The figure shows three views and two pictorial views of one solid part (mm, origin at its lowest corner). Answer the questions. A direction names the side the tool comes from. Coordinates: 2 decimals unless noted, no trailing zeros. Write each loop counter-clockwise with the first axis right and the second up, starting at its lowest first coordinate (ties: lowest second). Pieces come first, ordered by that corner, then holes. Notation, with made-up numbers: M 21.25,52.5 L 37.25,52.5 A23 ccw 37.25,67.5 Z; hole C 35.5,-12.5 d3. An arc over 180 degrees is marked long. Use a Markdown table: item, result. Add a question column.
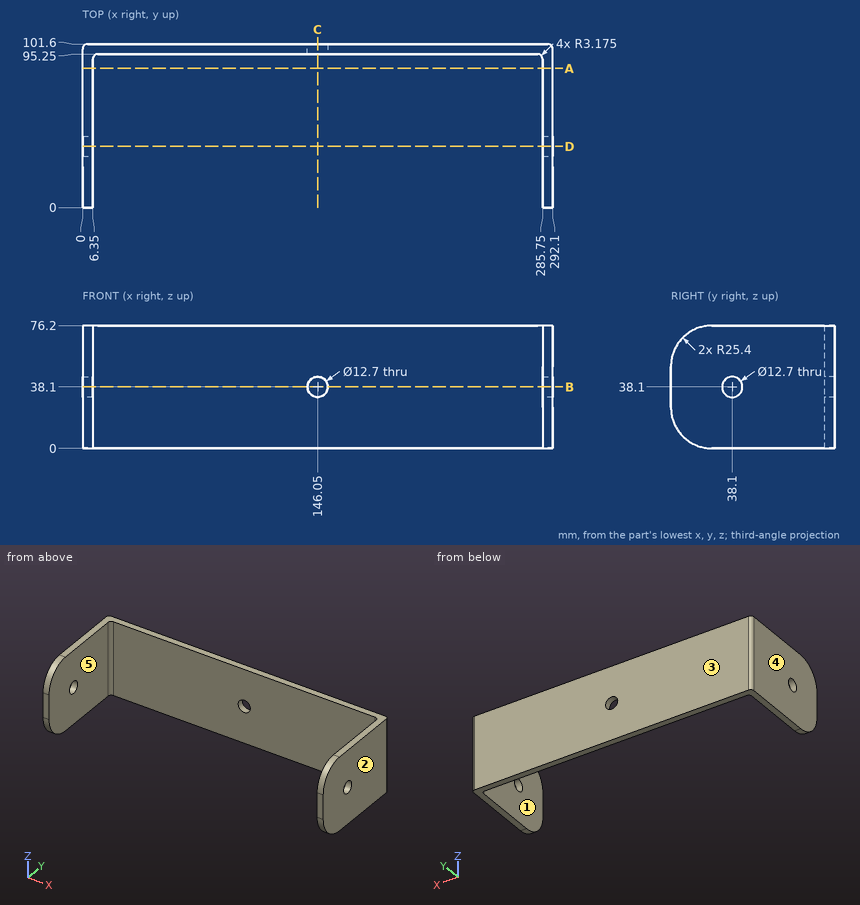
Item 1: Consider probe 1 along X at (y, z) = (92, 46.5); probe 2 along Z at (x, y) = (290, 38); probe 3 along Y at (x, z) = (287.75, 38.1). Determine where each line is inside the solid, lowest interval first.
Item 2: Determine the mould class of the marked faces 3, 4 and 5 for opening direction X: pulls with the +X half, pulls with the -X half, needs draft (parallel to the pull), parting line crosses it, or undercut.
Item 3: Find section C-C on x = 146.05. Give the vertices of the cut face in (y, z), then the cut area to 3 significant figures.
Item 4: Each of these flat-tipped pins is pushed along its axis until it touches: pin 1 (1 mm diameter, centred on x = 228.5, z = 63.5, fed in from -Y); pin 2 (16.5 mm diameter, centred on y = 38.1, z = 38.1, fed in from -X). Where does it stop, or does it pass through?
Item 5: For the marked faces 1 and 2, determine the directions among +Z, -Z, +X, -X, +Y, -Y from which every point of the face is accessible in a straight line to the end or side of a thin tool.
Item 6: Find section B-B on z = 38.1. Give the vertices of the cut face in (x, y) (3 decimals).
Item 7: Find section D-D on y = 38.1. Give the vertices of the cut face in (x, z), then the cut area to 3 significant figures.
Item 8: Find section A-A on y = 86.5. Give the vertices of the cut face in (x, z), then the cut area to 3 significant figures.
Geometry says:
| question | item | result |
|---|---|---|
| 1 | probe 1 | x = 0 to 6.35, 285.75 to 292.1 |
| 1 | probe 2 | z = 0 to 31.75, 44.45 to 76.2 |
| 1 | probe 3 | y = 0 to 31.75, 44.45 to 101.6 |
| 2 | face 3 | needs draft |
| 2 | face 4 | pulls with the -X half |
| 2 | face 5 | undercut |
| 3 | outline | M 95.25,0 L 101.6,0 L 101.6,31.75 L 95.25,31.75 Z; M 95.25,44.45 L 101.6,44.45 L 101.6,76.2 L 95.25,76.2 Z |
| 3 | area | 403 mm2 |
| 4 | pin 1 | stops at y = 95.25 |
| 4 | pin 2 | stops at x = 0 |
| 5 | face 1 | +Z, -Z, -Y |
| 5 | face 2 | +Z, -Z, +X, +Y, -Y |
| 6 | outline | M 0,0 L 6.35,0 L 6.35,31.75 L 0,31.75 Z; M 0,44.45 L 6.35,44.45 L 6.35,92.075 A3.175 cw 9.525,95.25 L 139.7,95.25 L 139.7,101.6 L 3.175,101.6 A3.175 ccw 0,98.425 Z; M 152.4,95.25 L 282.575,95.25 A3.175 cw 285.75,92.075 L 285.75,44.45 L 292.1,44.45 L 292.1,98.425 A3.175 ccw 288.925,101.6 L 152.4,101.6 Z; M 285.75,0 L 292.1,0 L 292.1,31.75 L 285.75,31.75 Z |
| 7 | outline | M 0,0 L 6.35,0 L 6.35,31.75 L 0,31.75 Z; M 0,44.45 L 6.35,44.45 L 6.35,76.2 L 0,76.2 Z; M 285.75,0 L 292.1,0 L 292.1,31.75 L 285.75,31.75 Z; M 285.75,44.45 L 292.1,44.45 L 292.1,76.2 L 285.75,76.2 Z |
| 7 | area | 806 mm2 |
| 8 | outline | M 0,0 L 6.35,0 L 6.35,76.2 L 0,76.2 Z; M 285.75,0 L 292.1,0 L 292.1,76.2 L 285.75,76.2 Z |
| 8 | area | 968 mm2 |
